Design review of the part built by this model. Coordinates are the model's own, in mm. Coordinates: 2 decimals unless noted, no trailing zeros. Write each loop counter-clockwise with the first axis right and the second up, starting at its lowest first coordinate (ties: lowest second). Pieces come first, ordered by that corner, then holes. Notation, with made-up numbers: (40.5, -9) - (88.5, -9) arc R21 cw to (88.5, -1) - close; hole circle Ø9 at (-5, 62). An arc over 180 degrees is marked (long way). One line per item, written item: value.
from build123d import *

# Parameters (mm, degrees)
SKETCH1_R                = 88
BOSS_EXTRUDE3_DEPTH      = 25
SKETCH4_W                = 10.4719
SKETCH4_H                = 13.351164338
BOSS_EXTRUDE4_DEPTH      = 25
FILLET2_R                = 4
CIRPATTERN1_COUNT        = 30
FILLET2_OF_CIRPATTERN1_R = 4
SKETCH6_R                = 10
BOSS_EXTRUDE5_DEPTH      = 60
BOSS_EXTRUDE6_START      = 10
SKETCH7_R                = 10
BOSS_EXTRUDE6_DEPTH      = 10
SKETCH8_R                = 10
BOSS_EXTRUDE7_DEPTH      = 10
SKETCH9_R                = 10
BOSS_EXTRUDE8_DEPTH      = 25
SKETCH10_R               = 10
BOSS_EXTRUDE9_DEPTH      = 42.5
SKETCH12_R               = 12.5
CUT_EXTRUDE1_DEPTH       = 12
CUT_EXTRUDE2_START       = -55.5
SKETCH13_R               = 10
CUT_EXTRUDE2_DEPTH       = 55.5
SKETCH14_R               = 10
BOSS_EXTRUDE10_DEPTH     = 440
SKETCH15_R               = 105
BOSS_EXTRUDE12_DEPTH     = 25
BOSS_EXTRUDE13_START     = 30
SKETCH16_R               = 105
BOSS_EXTRUDE13_DEPTH     = 30
SKETCH17_R               = 10
BOSS_EXTRUDE14_DEPTH     = 50
CUT_EXTRUDE3_START       = -700
SKETCH18_R               = 10
CUT_EXTRUDE3_DEPTH       = 700


with BuildPart() as part:
    # Sketch1 → Boss-Extrude3 (new body)
    with BuildSketch(Plane.XY):
        Circle(SKETCH1_R)
    extrude(amount=BOSS_EXTRUDE3_DEPTH)

    # Sketch4 → Boss-Extrude4 (add)
    with BuildSketch(Plane.XY.offset(25)):
        with Locations((0, 93.324417831)):
            Rectangle(SKETCH4_W, SKETCH4_H)
    boss_extrude4 = extrude(amount=-BOSS_EXTRUDE4_DEPTH)

    # Fillet2
    fillet2_edges = [part.edges().sort_by_distance(p)[0] for p in [
        (5.23595, 100, 12.5),
        (0, 100, 0),
        (-5.23595, 100, 12.5),
        (0, 100, 25),
    ]]
    fillet(fillet2_edges, radius=FILLET2_R)

    # CirPattern1: Boss-Extrude4 ×30 about axis
    cirpattern1_axis = Axis((0, 0.317667884, 0), (0, 0, 1))
    for i in range(1, CIRPATTERN1_COUNT):
        add(boss_extrude4.rotate(cirpattern1_axis, i * 360 / CIRPATTERN1_COUNT))

    # Fillet2 of CirPattern1
    fillet2_of_cirpattern1_edges = [part.edges().sort_by_distance(p)[0] for p in [
        (-15.603590285, 98.910317096, 12.5),
        (-20.725122215, 97.821701879, 0),
        (-25.846654145, 96.733086661, 12.5),
        (-20.725122215, 97.821701879, 25),
        (-35.7611788, 93.511662322, 12.5),
        (-40.544457139, 91.382009596, 0),
        (-45.327735478, 89.252356869, 12.5),
        (-40.544457139, 91.382009596, 25),
        (-54.3558322, 84.039982796, 12.5),
        (-58.591804732, 80.962368605, 0),
        (-62.827777264, 77.884754413, 12.5),
        (-58.591804732, 80.962368605, 25),
        (-70.574874905, 70.909236365, 12.5),
        (-74.078409304, 67.018167216, 0),
        (-77.581943702, 63.127098067, 12.5),
        (-74.078409304, 67.018167216, 25),
        (-83.709456921, 54.693299655, 12.5),
        (-86.327431921, 50.158833942, 0),
        (-88.945406921, 45.624368229, 12.5),
        (-86.327431921, 50.158833942, 25),
        (-93.185533987, 36.100886913, 12.5),
        (-94.803531519, 31.121202547, 0),
        (-96.42152905, 26.14151818, 12.5),
        (-94.803531519, 31.121202547, 25),
        (-98.588956064, 15.944575793, 12.5),
        (-99.136261871, 10.737308875, 0),
        (-99.683567678, 5.530041957, 12.5),
        (-99.136261871, 10.737308875, 25),
        (-99.683567678, -4.894706189, 12.5),
        (-99.136261871, -10.101973107, 0),
        (-98.588956064, -15.309240025, 12.5),
        (-99.136261871, -10.101973107, 25),
        (-96.42152905, -25.506182413, 12.5),
        (-94.803531519, -30.485866779, 0),
        (-93.185533987, -35.465551145, 12.5),
        (-94.803531519, -30.485866779, 25),
        (-88.945406921, -44.989032461, 12.5),
        (-86.327431921, -49.523498174, 0),
        (-83.709456921, -54.057963887, 12.5),
        (-86.327431921, -49.523498174, 25),
        (-77.581943702, -62.491762299, 12.5),
        (-74.078409304, -66.382831448, 0),
        (-70.574874905, -70.273900597, 12.5),
        (-74.078409304, -66.382831448, 25),
        (-62.827777264, -77.249418645, 12.5),
        (-58.591804732, -80.327032837, 0),
        (-54.3558322, -83.404647029, 12.5),
        (-58.591804732, -80.327032837, 25),
        (-45.327735478, -88.617021102, 12.5),
        (-40.544457139, -90.746673828, 0),
        (-35.7611788, -92.876326554, 12.5),
        (-40.544457139, -90.746673828, 25),
        (-25.846654145, -96.097750894, 12.5),
        (-20.725122215, -97.186366111, 0),
        (-15.603590285, -98.274981329, 12.5),
        (-20.725122215, -97.186366111, 25),
        (-5.23595, -99.364664232, 12.5),
        (0, -99.364664232, 0),
        (5.23595, -99.364664232, 12.5),
        (0, -99.364664232, 25),
        (15.603590285, -98.274981329, 12.5),
        (20.725122215, -97.186366111, 0),
        (25.846654145, -96.097750894, 12.5),
        (20.725122215, -97.186366111, 25),
        (35.7611788, -92.876326554, 12.5),
        (40.544457139, -90.746673828, 0),
        (45.327735478, -88.617021102, 12.5),
        (40.544457139, -90.746673828, 25),
        (54.3558322, -83.404647029, 12.5),
        (58.591804732, -80.327032837, 0),
        (62.827777264, -77.249418645, 12.5),
        (58.591804732, -80.327032837, 25),
        (70.574874905, -70.273900597, 12.5),
        (74.078409304, -66.382831448, 0),
        (77.581943702, -62.491762299, 12.5),
        (74.078409304, -66.382831448, 25),
        (83.709456921, -54.057963887, 12.5),
        (86.327431921, -49.523498174, 0),
        (88.945406921, -44.989032461, 12.5),
        (86.327431921, -49.523498174, 25),
        (93.185533987, -35.465551145, 12.5),
        (94.803531519, -30.485866779, 0),
        (96.42152905, -25.506182413, 12.5),
        (94.803531519, -30.485866779, 25),
        (98.588956064, -15.309240025, 12.5),
        (99.136261871, -10.101973107, 0),
        (99.683567678, -4.894706189, 12.5),
        (99.136261871, -10.101973107, 25),
        (99.683567678, 5.530041957, 12.5),
        (99.136261871, 10.737308875, 0),
        (98.588956064, 15.944575793, 12.5),
        (99.136261871, 10.737308875, 25),
        (96.42152905, 26.14151818, 12.5),
        (94.803531519, 31.121202547, 0),
        (93.185533987, 36.100886913, 12.5),
        (94.803531519, 31.121202547, 25),
        (88.945406921, 45.624368229, 12.5),
        (86.327431921, 50.158833942, 0),
        (83.709456921, 54.693299655, 12.5),
        (86.327431921, 50.158833942, 25),
        (77.581943702, 63.127098067, 12.5),
        (74.078409304, 67.018167216, 0),
        (70.574874905, 70.909236365, 12.5),
        (74.078409304, 67.018167216, 25),
        (62.827777264, 77.884754413, 12.5),
        (58.591804732, 80.962368605, 0),
        (54.3558322, 84.039982796, 12.5),
        (58.591804732, 80.962368605, 25),
        (45.327735478, 89.252356869, 12.5),
        (40.544457139, 91.382009596, 0),
        (35.7611788, 93.511662322, 12.5),
        (40.544457139, 91.382009596, 25),
        (25.846654145, 96.733086661, 12.5),
        (20.725122215, 97.821701879, 0),
        (15.603590285, 98.910317096, 12.5),
        (20.725122215, 97.821701879, 25),
    ]]
    fillet(fillet2_of_cirpattern1_edges, radius=FILLET2_OF_CIRPATTERN1_R)

    # Sketch6 → Boss-Extrude5 (add)
    with BuildSketch(Plane.XY.offset(25)):
        Circle(SKETCH6_R)
    extrude(amount=BOSS_EXTRUDE5_DEPTH)

    # Sketch7 → Boss-Extrude6 (add)
    with BuildSketch(Plane(origin=(0, 0, 0), x_dir=(-1, 0, 0), z_dir=(0, 0, -1)).offset(BOSS_EXTRUDE6_START)):
        with Locations(Location((0, 0, 0), (0, 0, 180))):
            Circle(SKETCH7_R)
    extrude(amount=-BOSS_EXTRUDE6_DEPTH)

    # Sketch8 → Boss-Extrude7 (add)
    with BuildSketch(Plane.XY.offset(85)):
        Circle(SKETCH8_R)
    extrude(amount=BOSS_EXTRUDE7_DEPTH)

    # Sketch9 → Boss-Extrude8 (add)
    with BuildSketch(Plane.XY.offset(95)):
        Circle(SKETCH9_R)
    extrude(amount=BOSS_EXTRUDE8_DEPTH)

    # Sketch10 → Boss-Extrude9 (add)
    with BuildSketch(Plane.XY.offset(120)):
        Circle(SKETCH10_R)
    extrude(amount=BOSS_EXTRUDE9_DEPTH)

    # Sketch12 → Cut-Extrude1 (cut)
    with BuildSketch(Plane.XY.offset(162.5)):
        Circle(SKETCH12_R)
    extrude(amount=-CUT_EXTRUDE1_DEPTH, mode=Mode.SUBTRACT)

    # Sketch13 → Cut-Extrude2 (cut)
    with BuildSketch(Plane.XY.offset(150.5).offset(CUT_EXTRUDE2_START)):
        Circle(SKETCH13_R)
    extrude(amount=CUT_EXTRUDE2_DEPTH, mode=Mode.SUBTRACT)

    # Sketch14 → Boss-Extrude10 (add)
    with BuildSketch(Plane.XY.offset(95)):
        Circle(SKETCH14_R)
    extrude(amount=BOSS_EXTRUDE10_DEPTH)

    # Sketch15 → Boss-Extrude12 (add)
    with BuildSketch(Plane(origin=(0, 0, 0), x_dir=(-1, 0, 0), z_dir=(0, 0, -1))):
        Circle(SKETCH15_R)
    extrude(amount=-BOSS_EXTRUDE12_DEPTH)

    # Sketch16 → Boss-Extrude13 (add)
    with BuildSketch(Plane(origin=(0, 0, 0), x_dir=(-1, 0, 0), z_dir=(0, 0, -1)).offset(BOSS_EXTRUDE13_START)):
        Circle(SKETCH16_R)
    extrude(amount=-BOSS_EXTRUDE13_DEPTH)

    # Sketch17 → Boss-Extrude14 (add)
    with BuildSketch(Plane.XY.offset(535)):
        Circle(SKETCH17_R)
    extrude(amount=BOSS_EXTRUDE14_DEPTH)

    # Sketch18 → Cut-Extrude3 (cut)
    with BuildSketch(Plane.XY.offset(585).offset(CUT_EXTRUDE3_START)):
        Circle(SKETCH18_R)
    extrude(amount=CUT_EXTRUDE3_DEPTH, mode=Mode.SUBTRACT)


solid = part.part
1. Insertion check: pin 1 Ø6 at (y, z) = (-6, 1) entering from -X; pin 2 Ø4 at (x, z) = (47, -5) entering from +Y; pin 3 Ø1 at (y, z) = (-19.5, 5.5) entering from +X; pin 4 Ø23 at (x, y) = (0, 0) entering from +Z. Each pin has a flat end and moves straight along its axis. Give the tip position at first contact, or say it passes through.
Answer block:
pin 1: stops at x = -104.96
pin 2: stops at y = 94.87
pin 3: stops at x = 103.27
pin 4: stops at z = 25
2. Consider section C-C, the plane z = 8. Write out the cut boundary in (x, y), then the cut area to 3 significant figures.
Answer block:
outline: circle Ø210 at (0, 0); hole circle Ø20 at (0, 0)
area: 34,300 mm^2
3. Consider section A-A, the plane y = 0. Write out the cut boundary in (x, z), then the cut area to 4 significant figures.
Answer block:
outline: (-105, -30) - (-10, -30) - (-10, 25) - (-105, 25) - close; (10, -30) - (105, -30) - (105, 25) - (10, 25) - close
area: 10,450 mm^2
4. Consider section D-D, the plane y = -28. Write out the cut boundary in (x, z), then the cut area to 3 significant figures.
Answer block:
outline: (-101.2, -30) - (101.2, -30) - (101.2, 25) - (-101.2, 25) - close
area: 11,100 mm^2
5. Wall thickness on line 1 along Y through (x, z) = (0, -17.5); line 2 along Y through (x, z) = (18, 3.5); line 3 along X through (y, z) = (-20, 6.5): over which ranges is each line inside the solid? List them lowest first.
Answer block:
line 1: y = -105 to -10, 10 to 105
line 2: y = -103.45 to 103.45
line 3: x = -103.08 to 103.08
6. Mouldability with a two-part tool opening along X and no side actions: class faces 1 (the face through (1, -22, -30)), 2 (the face through (-2.17, -9.76, -2.89)), 3 (the face through (-100.15, 31.54, -2.89)) as released by +X, released by -X, zero draft, split by the parting line, or undercut.
Answer block:
face 1: zero draft
face 2: undercut
face 3: split by the parting line
